Source: CAD feature listing. Evaluate the final solid. Frame: model axes, mm. A direction names the side the tool comes from. Give positions to 0.01 mm unless a question says otherwise; leave off trailing zeros. Loops run counter-clockwise (first coordinate to the right, second up) from the corner with the lowest first, then second, coordinate; pieces in that order, holes last. Notation, with made-up numbers: M 4.5,-1.5 L 35.5,-1.5 A13 ccw 35.5,21.5 Z; hole C 83.25,-16 d1. An arc over 180 degrees is marked long. Answer in a Markdown table with one row per item.
```python
from build123d import *

# Parameters (mm, degrees)
SKETCH1_R               = 1.5
BOSS_EXTRUDE1_DEPTH     = 6
SKETCH3_W               = 13
SKETCH3_H               = 23
SKETCH3_W_2             = 9.027129354
SKETCH3_H_2             = 6.528275522
CUT_EXTRUDE1_DEPTH      = 14
FILLET1_R               = 1
BOSS_EXTRUDE4_DEPTH     = 120
SKETCH7_W               = 4
SKETCH7_H               = 6
CUT_EXTRUDE5_DEPTH      = 15
SKETCH8_R               = 10
BOSS_EXTRUDE5_DEPTH     = 2
CUT_EXTRUDE6_DEPTH      = 18
FILLET4_R               = 2
FILLET5_R               = 5
CUT_EXTRUDE8_DEPTH      = 20
CUT_EXTRUDE8_DEPTH_BACK = 20
CUT_EXTRUDE9_DEPTH      = 20
CUT_EXTRUDE9_DEPTH_BACK = 20
BOSS_EXTRUDE9_DEPTH     = 6
SKETCH16_R              = 10
BOSS_EXTRUDE10_DEPTH    = 2
FILLET6_R               = 5


with BuildPart() as part:
    # Sketch1 → Boss-Extrude1 (new body)
    with BuildSketch(Plane(origin=(0, 0, 0), x_dir=(1, 0, 0), z_dir=(0, 1, 0))):
        with BuildLine():
            Line((-10, 20), (-10, -100))
            Line((-10, -100), (10, -100))
            Line((10, -100), (10, 20))
            ThreePointArc((10, 20), (0, 30), (-10, 20))
        make_face()
        with Locations(Location((0, 0, 0), (0, 0, 270))):
            Circle(SKETCH1_R, mode=Mode.SUBTRACT)
        with Locations(Location((0, 20, 0), (0, 0, 270))):
            Circle(SKETCH1_R, mode=Mode.SUBTRACT)
    extrude(amount=BOSS_EXTRUDE1_DEPTH)

    # Sketch3 → Cut-Extrude1 (cut)
    with BuildSketch(Plane(origin=(0, 6, 0), x_dir=(1, 0, 0), z_dir=(0, 1, 0))):
        Polygon((7, -7), (-7, -7), (0, -27), align=None)
        Polygon((7, -62), (-7, -62), (0, -32), align=None)
        with Locations((0, -83.5)):
            Rectangle(SKETCH3_W, SKETCH3_H)
        with Locations((0, 10)):
            Rectangle(SKETCH3_W_2, SKETCH3_H_2)
    extrude(amount=-CUT_EXTRUDE1_DEPTH, mode=Mode.SUBTRACT)

    # Fillet1
    fillet1_edges = [part.edges().sort_by_distance(p)[0] for p in [
        (-6.5, 3, 95),
        (-6.5, 3, 72),
        (6.5, 3, 72),
        (6.5, 3, 95),
        (0, 3, 32),
        (7, 3, 62),
        (-7, 3, 62),
        (-7, 3, 7),
        (7, 3, 7),
        (0, 3, 27),
        (-4.513564677, 3, -13.264137761),
        (4.513564677, 3, -13.264137761),
        (4.513564677, 3, -6.735862239),
        (-4.513564677, 3, -6.735862239),
    ]]
    fillet(fillet1_edges, radius=FILLET1_R)

    # Sketch6 → Boss-Extrude4 (add)
    with BuildSketch(Plane.XY.offset(100)):
        Polygon((14, 6), (10, 6), (10, 5), (12, 5), (12, 1), (10, 1), (10, 0), (14, 0), align=None)
    extrude(amount=-BOSS_EXTRUDE4_DEPTH)

    # Sketch7 → Cut-Extrude5 (cut)
    with BuildSketch(Plane.XY.offset(100)):
        with Locations((12, 3)):
            Rectangle(SKETCH7_W, SKETCH7_H)
    extrude(amount=-CUT_EXTRUDE5_DEPTH, mode=Mode.SUBTRACT)

    # Sketch8 → Boss-Extrude5 (add)
    with BuildSketch(Plane.XY.offset(100)):
        with Locations((0, 3)):
            Circle(SKETCH8_R)
    extrude(amount=BOSS_EXTRUDE5_DEPTH)

    # Sketch9 → Cut-Extrude6 (cut)
    with BuildSketch(Plane(origin=(0, 6, 0), x_dir=(1, 0, 0), z_dir=(0, 1, 0))):
        Polygon((10, 20), (14, 16), (14, 20), align=None)
        Polygon((10, -85), (14, -76.582524272), (14, -85), align=None)
    extrude(amount=-CUT_EXTRUDE6_DEPTH, mode=Mode.SUBTRACT)

    # Fillet4
    fillet4_edges = [part.edges().sort_by_distance(p)[0] for p in [
        (14, 3, -16),
    ]]
    fillet(fillet4_edges, radius=FILLET4_R)

    # Fillet5
    # the kernel refuses this fillet: 5 mm, written as the material it adds along each edge
    with BuildSketch(Plane(origin=(22.039392014, 6, 100), x_dir=(0, 0, -1), z_dir=(-1, 0, 0))) as fillet5_piece_1_section:
        with BuildLine():
            CenterArc((FILLET5_R, -FILLET5_R), FILLET5_R, 90, 90)
            Line((0, -FILLET5_R), (0, 0))
            Line((0, 0), (FILLET5_R, 0))
        make_face()
    fillet5_piece_1 = extrude(amount=44.078784028, mode=Mode.PRIVATE)
    fillet5_piece_1 = fillet5_piece_1 & Plane(origin=(0, 3, 98.854598336), x_dir=(1, 0, 0), z_dir=(0, 0, -1)) * Cylinder(10, 109, mode=Mode.PRIVATE)
    add(fillet5_piece_1)
    with BuildSketch(Plane(origin=(22.039392014, 0, 100), x_dir=(0, 0, -1), z_dir=(-1, 0, 0))) as fillet5_piece_2_section:
        with BuildLine():
            CenterArc((FILLET5_R, FILLET5_R), FILLET5_R, 180, 90)
            Line((0, FILLET5_R), (0, 0))
            Line((0, 0), (FILLET5_R, 0))
        make_face()
    fillet5_piece_2 = extrude(amount=44.078784028, mode=Mode.PRIVATE)
    fillet5_piece_2 = fillet5_piece_2 & Plane(origin=(0, 3, 98.854598336), x_dir=(1, 0, 0), z_dir=(0, 0, -1)) * Cylinder(10, 109, mode=Mode.PRIVATE)
    add(fillet5_piece_2)

    # Sketch13 → Cut-Extrude8 (cut, two sides: drawn at the far end of the back side and taken through both)
    with BuildSketch(Plane.XZ.offset(-CUT_EXTRUDE8_DEPTH_BACK)):
        with BuildLine():
            Line((-6.5, 73.5), (0, 80))
            Line((0, 80), (6.5, 86.5))
            Line((6.5, 86.5), (6.5, 94))
            ThreePointArc((6.5, 94), (6.207106781, 94.707106781), (5.5, 95))
            Line((5.5, 95), (9.539392014, 95))
            Line((9.539392014, 95), (9.539392014, 100))
            Line((9.539392014, 100), (10, 100))
            Line((10, 100), (10, 90))
            Line((10, 90), (14.142135624, 94.142135624))
            Line((14.142135624, 94.142135624), (18.212490394, 115.492902619))
            Line((18.212490394, 115.492902619), (-15.568958515, 115.492902619))
            Line((-15.568958515, 115.492902619), (-15.568958515, 64.431041485))
            Line((-15.568958515, 64.431041485), (-10, 70))
            Line((-10, 70), (-10, 100))
            Line((-10, 100), (-9.539392014, 100))
            Line((-9.539392014, 100), (-9.539392014, 95))
            Line((-9.539392014, 95), (-5.5, 95))
            ThreePointArc((-5.5, 95), (-6.207106781, 94.707106781), (-6.5, 94))
            Line((-6.5, 94), (-6.5, 73.5))
        make_face()
    extrude(amount=CUT_EXTRUDE8_DEPTH + CUT_EXTRUDE8_DEPTH_BACK, mode=Mode.SUBTRACT)

    # Sketch14 → Cut-Extrude9 (cut, two sides: drawn at the far end of the back side and taken through both)
    with BuildSketch(Plane.XZ.offset(-CUT_EXTRUDE9_DEPTH_BACK)):
        Polygon((0, 80), (19.360707344, 99.360707344), (19.360707344, 111.570074628), (-16.85715032, 110.200384013), (-16.85715032, 63.14284968), align=None)
    extrude(amount=CUT_EXTRUDE9_DEPTH + CUT_EXTRUDE9_DEPTH_BACK, mode=Mode.SUBTRACT)

    # Sketch15 → Boss-Extrude9 (add)
    with BuildSketch(Plane.XZ):
        Polygon((14.142135624, 94.142135624), (16.263884736, 92.020386512), (10, 85.756501776), (-10, 65.756501776), (-10, 74.242640687), (12.02081528, 96.263455967), align=None)
    extrude(amount=-BOSS_EXTRUDE9_DEPTH)

    # Sketch16 → Boss-Extrude10 (add)
    with BuildSketch(Plane(origin=(54.142135624, 0, 54.142135624), x_dir=(0.7071067811865469, 0, -0.7071067811865481), z_dir=(0.7071067811865481, 0, 0.7071067811865469))):
        with Locations((-56.56823931, 3)):
            Circle(SKETCH16_R)
    extrude(amount=BOSS_EXTRUDE10_DEPTH)

    # Fillet6
    fillet6_edges = [part.edges().sort_by_distance(p)[0] for p in [
        (-10, 3, 74.242640687),
    ]]
    fillet(fillet6_edges, radius=FILLET6_R)


solid = part.part
```
1) Section C-C, the plane z = 38.5. Return loops of the section in (x, y), then the cut area to 3 significant figures.
Reply:
| item | result |
|---|---|
| outline | M -10,0 L -1.52,0 L -1.52,6 L -10,6 Z; M 1.52,0 L 14,0 L 14,6 L 1.52,6 Z; hole M 10,1 L 12,1 L 12,5 L 10,5 Z |
| area | 118 mm² |
2) Pull-direction query (Z, two-part tool) for faces 1 (the flat face through (-10, 3, 25)), 2 (the flat face through (13.088, 2.958, 88.845)), 3 (the cylindrical face through (9.63, 9.76, 100.05)), 4 (the flat face through (4.514, 3, -10)); classes: released by +Z, released by -Z, zero draft, split by the parting line, or undercut.
Reply:
| item | result |
|---|---|
| face 1 | zero draft |
| face 2 | undercut |
| face 3 | split by the parting line |
| face 4 | undercut |
3) Material intervals for L1, parallel to X at y = 3.3, z = -20; L2, parallel to X at y = 2, z = 34; L3, parallel to X at y = 2.25, z = 58.5, sorted ascending.
Reply:
| item | result |
|---|---|
| L1 | x = -10 to -1.5, 1.5 to 10 |
| L2 | x = -10 to 10, 12 to 14 |
| L3 | x = -10 to -6.18, 6.18 to 10, 12 to 14 |
4) Pin query (flat end, axial travel): pin 1 Ø5 at (y, z) = (1.5, 45) entering from +X; pin 2 Ø12 at (x, z) = (-2, 15) entering from +Y; pin 3 Ø5 at (x, y) = (13, 1) entering from +Z; pin 4 Ø6 at (y, z) = (10, 64.5) entering from +X. Return the tip coordinate at first contact, or that it passes through.
Reply:
| item | result |
|---|---|
| pin 1 | stops at x = 14 |
| pin 2 | stops at y = 6 |
| pin 3 | stops at z = 100.61 |
| pin 4 | passes through |
5) Section A-A, the plane z = 0. Return loops of the section in (x, y).
Reply:
| item | result |
|---|---|
| outline | M -10,0 L -1.5,0 L -1.5,6 L -10,6 Z; M 1.5,0 L 14,0 L 14,6 L 1.5,6 Z; hole M 10,1 L 12,1 L 12,5 L 10,5 Z |
6) Section B-B, the plane z = 66.5. Return loops of the section in (x, y), then the cut area to 3 significant figures.
Reply:
| item | result |
|---|---|
| outline | M -10,0 L 14,0 L 14,6 L -10,6 Z; hole M 10,1 L 12,1 L 12,5 L 10,5 Z |
| area | 136 mm² |
7) Set-up query: faces 5 (the flat face through (15.458, 3.14, 95.655)), 6 (the flat face through (14, 3, 31)), 7 (the flat face through (1.6, 2.96, 85.84)), 8 (the flat face through (0, 3, 62)). Return all of +Z, -Z, +X, -X, +Y, -Y with unobstructed straight access to the full face (end or side cutting, diameter ignored); none if empty.
Reply:
| item | result |
|---|---|
| face 5 | +Z, +X, +Y, -Y |
| face 6 | -Z, +X, +Y, -Y |
| face 7 | -X, +Y, -Y |
| face 8 | +Y, -Y |
